from build123d import *

# Parameters (mm, degrees)
CUT_EXTRUDE_1_DEPTH      = 23
CUT_EXTRUDE_1_DEPTH_BACK = 3
SKETCH_8_R               = 1.5
THREAD_2_PITCH           = 0.3175
SKETCH_9_R               = 5
CUT_EXTRUDE_2_DEPTH      = 15


with BuildPart() as part:
    # 扫描1: sweep along a path in 草图7
    with BuildLine(Plane(origin=(0, 20, 0), x_dir=(1, 0, 0), z_dir=(0, 1, 0))) as sweep_1_path:
        CenterArc((0, 0), 8.222167991, 0, 360)
    # 草图6 → 扫描1 (sweep)
    with BuildSketch(Plane.XY):
        Polygon((0, 0), (0, 98), (5, 98), (5, 73), (10, 73), (10, 72), (22, 72), (22, 31.681513685), (21, 31.681513685), (21, 30.681513685), (22, 30.681513685), (22, 2.337983279), (21.5, 1.837983279), (5, 1.837983279), (5, 0), align=None)
    sweep(path=sweep_1_path.line)

    # 草图8 → 切除-拉伸1 (cut, two sides: drawn at the far end of the back side and taken through both)
    with BuildSketch(Plane.XY.offset(-CUT_EXTRUDE_1_DEPTH_BACK)):
        with Locations(Location((0, 90.222635434, 0), (0, 0, 270))):
            Circle(SKETCH_8_R)
    extrude(amount=CUT_EXTRUDE_1_DEPTH + CUT_EXTRUDE_1_DEPTH_BACK, mode=Mode.SUBTRACT)

    # 螺纹线2: the profile of 螺纹线轮廓3 profile screwed along a right-hand helix of 23.622047 turns, 6 arcs to a turn; built about Z, then put on its axis
    thread_2_z = Axis((0, 0, 0), (0, 0, 1))
    thread_2_corners = [(1.5003, 0, -0.000173205), (1.5003, 0, 0.277985704), (1.328148085, 0, 0.17859375), (1.328148085, 0, 0.09921875)]
    with BuildLine(mode=Mode.PRIVATE) as thread_2_profile:
        Line(thread_2_corners[0], thread_2_corners[1])
        Line(thread_2_corners[1], thread_2_corners[2])
        Line(thread_2_corners[2], thread_2_corners[3])
        Line(thread_2_corners[3], thread_2_corners[0])
    thread_2_cap = Face(thread_2_profile.wire())
    thread_2_turn_angles = [0, 30, 60, 90, 120, 150, 180, 210, 240, 270, 300, 330, 360]
    thread_2_turn_weights = [1, 0.8660254037844387, 1, 0.8660254037844387, 1, 0.8660254037844387, 1, 0.8660254037844387, 1, 0.8660254037844387, 1, 0.8660254037844387, 1]
    thread_2_turn_rails = [Edge.make_bspline([Vector(p[0], p[1], 0).rotate(thread_2_z, thread_2_turn_angles[k]) / thread_2_turn_weights[k] + Vector(0, 0, p[2] + THREAD_2_PITCH * thread_2_turn_angles[k] / 360) for k in range(13)], [0, 0, 0, 1, 1, 2, 2, 3, 3, 4, 4, 5, 5, 6, 6, 6], 2, thread_2_turn_weights) for p in thread_2_corners]
    thread_2_turn_sides = [Face.make_surface_from_curves(thread_2_turn_rails[p[0]], thread_2_turn_rails[p[1]]) for p in [(0, 1), (1, 2), (2, 3), (3, 0)]]
    thread_2_last_angles = [8280, 8310, 8340, 8370, 8400, 8430, 8460, 8481.968503937, 8503.937007874]
    thread_2_last_weights = [1, 0.8660254037844387, 1, 0.8660254037844387, 1, 0.8660254037844387, 1, 0.9273896394584102, 1]
    thread_2_last_rails = [Edge.make_bspline([Vector(p[0], p[1], 0).rotate(thread_2_z, thread_2_last_angles[k]) / thread_2_last_weights[k] + Vector(0, 0, p[2] + THREAD_2_PITCH * thread_2_last_angles[k] / 360) for k in range(9)], [0, 0, 0, 1, 1, 2, 2, 3, 3, 4, 4, 4], 2, thread_2_last_weights) for p in thread_2_corners]
    thread_2_last_sides = [Face.make_surface_from_curves(thread_2_last_rails[p[0]], thread_2_last_rails[p[1]]) for p in [(0, 1), (1, 2), (2, 3), (3, 0)]]
    thread_2 = Plane(origin=(0, 90.222635434, -3), x_dir=(1, 0, 0), z_dir=(0, 0, 1)) * Solid(Shell([*[p.moved(Location((0, 0, THREAD_2_PITCH * i))) for i in range(23) for p in thread_2_turn_sides], *thread_2_last_sides, thread_2_cap, thread_2_cap.rotate(thread_2_z, 8503.937007874).moved(Location((0, 0, THREAD_2_PITCH * 8503.937007874 / 360)))]))
    add(thread_2)

    # 草图9 → 切除-拉伸2 (cut)
    with BuildSketch(Plane(origin=(0, 100, 0), x_dir=(1, 0, 0), z_dir=(0, 1, 0))):
        Circle(SKETCH_9_R)
    extrude(amount=-CUT_EXTRUDE_2_DEPTH, mode=Mode.SUBTRACT)


solid = part.part
For this review, take the finished solid that the model builds, in its own axes (mm). A direction names the side the tool comes from. Coordinates: 2 decimals unless noted, no trailing zeros. Loops run counter-clockwise (first coordinate to the right, second up) from the corner with the lowest first, then second, coordinate; pieces in that order, holes last. Notation, with made-up numbers: (19, 57.5) - (63, 57.5) arc R24 ccw to (63, 92.5) - close; hole circle Ø9 at (82.5, -19.5). An arc over 180 degrees is marked (long way). Return JSON: item names as keys, results as strings.
Item 1: For faces 1 (the cylindrical face through (-1.08, 79.08, 4.88)), 2 (the cylindrical face through (-4.769, 52.123, 21.477)), list the 3-axis set-ups (+Z, -Z, +X, -X, +Y, -Y) from which the entire face can be reached by the end or side of a thin tool; tool diameter is ignored.
Determined:
{"face 1": "+Y", "face 2": "+Y, -Y"}
Item 2: Take a section at A-A (y = 27). Give the boundary of the cut face in (x, z), then the cut area to 3 significant figures.
Determined:
{"outline": "circle Ø44 at (0, 0)", "area": "1,520 mm2"}
Item 3: Mouldability with a two-part tool opening along Y and no side actions: class faces 3 (the flat face through (0, 85, 0)), 4 (the cylindrical face through (-1.08, 0.93, 4.88)), 5 (the cylindrical face through (20.03, 31.19, -6.31)) as pulls with the +Y half, pulls with the -Y half, needs draft (parallel to the pull), parting line crosses it, or undercut.
Determined:
{"face 3": "pulls with the +Y half", "face 4": "needs draft", "face 5": "undercut"}
Item 4: Insertion check: pin 1 (1.5 mm diameter, centred on x = -15.5, y = 64.5, fed in from -Z); pin 2 (1 mm diameter, centred on x = 12.5, z = 12.5, fed in from -Y); pin 3 (4 mm diameter, centred on x = -1, y = 16, fed in from -Z); pin 4 (12 mm diameter, centred on y = 50, z = -0.5, fed in from -X). Each pin has a flat end and moves straight along its axis. Give the tip position at first contact, or say it passes through.
Determined:
{"pin 1": "stops at z = -16.32", "pin 2": "stops at y = 1.84", "pin 3": "stops at z = -22", "pin 4": "stops at x = -22"}
Item 5: For line 1 (Y direction, x = 7, z = 16); line 2 (X direction, y = 68.5, z = -0.5); line 3 (Y direction, x = -2.5, z = 5), list the stretches that pass through material, from the lowest coordinate up.
Determined:
{"line 1": "y = 1.84 to 72", "line 2": "x = -21.99 to 21.99", "line 3": "y = 1.84 to 73"}
